Autodesk Inventor part; units mm, degrees
ref_plane "YZ Plane" through (0, 0, 0) normal (1, 0, 0) x (0, 1, 0)
ref_plane "XZ Plane" through (0, 0, 0) normal (0, 1, 0) x (-1, 0, 0)
ref_plane "XY Plane" through (0, 0, 0) normal (0, 0, 1) x (1, 0, 0)
sketch "Sketch1" plane through (0, 0, 0) normal (0, 1, 0) x (-1, 0, 0)
  line L0 (0, 0) -> (15, 0)
  line L1 (15, 0) -> (15, -7)
  line L2 (15, -7) -> (0, -7)
  line L3 (0, -7) -> (0, 0)
  dimension "d0" = 15
  dimension "d1" = 7
extrude "Extrusion1" add sketch "Sketch1" along normal blind 10
sketch "Sketch2" plane through (0, 10, 0) normal (0, 1, 0) x (1, 0, 0)
  line L0 (-12.6158, 4.9907) -> (24.8842, 4.9907)
  line L1 (24.8842, 4.9907) -> (24.8842, 1.9907)
  line L2 (24.8842, 1.9907) -> (-12.6158, 1.9907)
  line L3 (-12.6158, 1.9907) -> (-12.6158, 4.9907)
  point P0 (0, 0)
  dimension "d4" = 37.5
  dimension "d5" = 3
extrude "Extrusion2" add sketch "Sketch2" along normal blind 0.98
sketch "Sketch3" plane through (0, 0, 0) normal (0, -1, 0) x (1, 0, 0)
  line L0 (-12.6158, -4.9907) -> (-12.6158, -1.9907)
  line L1 (0, -1.9907) -> (-12.6158, -1.9907)
  line L2 (-12.6158, -4.9907) -> (-11, -4.9907)
  line L3 (-11, -4.9907) -> (-11, -1.9907)
  line L4 (-11, -1.9907) -> (-12.6158, -1.9907)
  line L5 (-12.6158, -1.9907) -> (-12.6158, -4.9907)
  line L6 (-8, -4.9907) -> (-6.3079, -4.9907)
  line L7 (-6.3079, -4.9907) -> (-6.3079, -1.9907)
  line L8 (-6.3079, -1.9907) -> (-8, -1.9907)
  line L9 (-8, -1.9907) -> (-8, -4.9907)
  line L10 (-4, -4.9907) -> (-2, -4.9907)
  line L11 (-2, -4.9907) -> (-2, -1.9907)
  line L12 (-2, -1.9907) -> (-4, -1.9907)
  line L13 (-4, -1.9907) -> (-4, -4.9907)
  point P0 (0, 0)
extrude "Extrusion3" add sketch "Sketch3" along normal blind 5
properties part number "limit_switch"
Geometry check sheet. Reference: the model listing, model coordinates, mm. A direction names the side the tool comes from. Give positions to 0.01 mm unless a question says otherwise; leave off trailing zeros. Order: outer loops, then holes, each group sorted by start corner. A loop starts at its lowest first (then second) coordinate and runs counter-clockwise, first axis right, second up.
1. Release check for a two-part mould opening along X. For faces 5 (the face through (-6.308, -2, -4)), 6 (the face through (-15, 5, -3)), 7 (the face through (-7, 10, -6)) record: pulls with the +X half, pulls with the -X half, needs draft (parallel to the pull), parting line crosses it, or undercut.
2. Section check D-D, the plane y = 6. Enter the section's corners in (x, z), and give its area (3 significant figures).
3. Section check A-A, the plane y = -2.5. Enter the section's corners in (x, z), and give its area (3 significant figures).
4. Section check B-B, the plane z = -2.5. Enter the section's corners in (x, y).
5. Gauge pin test, flat ends, axial feed: pin 1 Ø0.9 at (y, z) = (-3.5, -4) entering from +X; pin 2 Ø0.6 at (x, y) = (-3.5, -3.5) entering from -Z; pin 3 Ø3.5 at (y, z) = (5.5, -5) entering from +X. Record the tip position at first contact, or that the pin passes through.
6. Access from +Z, -Z, +X, -X, +Y, -Y to the whole of each face (thin tool, end or side, straight path). Record for faces 1 (the face through (-7, -2, -4.991)), 2 (the face through (-12.616, 10.5, -3.5)), 3 (the face through (-8, -2, -3)), 4 (the face through (-2, -2, -4)).
7. Section check C-C, the plane x = 3.5. Enter the section's corners in (y, z).
8. Thickness scan on L1, parallel to X at y = -3.25, z = -4; L2, parallel to X at y = 1.75, z = -5.75; L3, parallel to Y at x = 17.5, z = -3.25. Record the ranges inside material, lowest first.
Values follow:
1. face 5: undercut
1. face 6: pulls with the -X half
1. face 7: needs draft
2. outline: (-15, -7) - (0, -7) - (0, 0) - (-15, 0) - close
2. area: 105 mm2
3. outline: (-12.62, -4.99) - (-11, -4.99) - (-11, -1.99) - (-12.62, -1.99) - close; (-8, -4.99) - (-6.31, -4.99) - (-6.31, -1.99) - (-8, -1.99) - close; (-4, -4.99) - (-2, -4.99) - (-2, -1.99) - (-4, -1.99) - close
3. area: 15.9 mm2
4. outline: (-15, 0) - (-12.62, 0) - (-12.62, -5) - (-11, -5) - (-11, 0) - (-8, 0) - (-8, -5) - (-6.31, -5) - (-6.31, 0) - (-4, 0) - (-4, -5) - (-2, -5) - (-2, 0) - (0, 0) - (0, 10) - (24.88, 10) - (24.88, 10.98) - (-12.62, 10.98) - (-12.62, 10) - (-15, 10) - close
5. pin 1: stops at x = -2
5. pin 2: stops at z = -4.99
5. pin 3: stops at x = 0
6. face 1: -Z, +X, -X, -Y
6. face 2: +Z, -Z, -X, +Y
6. face 3: +Z, -Z, -Y
6. face 4: +Z, -Z, +X, -Y
7. outline: (10, -4.99) - (10.98, -4.99) - (10.98, -1.99) - (10, -1.99) - close
8. L1: x = -12.62 to -11, -8 to -6.31, -4 to -2
8. L2: x = -15 to 0
8. L3: y = 10 to 10.98
